Autodesk Inventor part; units mm, degrees
ref_plane "Work Plane1" through (-76.2, 0, 0) normal (-1, 0, 0) x (0, 0, 1)
ref_plane "YZ Plane" through (0, 0, 0) normal (1, 0, 0) x (0, 1, 0)
ref_plane "XZ Plane" through (0, 0, 0) normal (0, 1, 0) x (-1, 0, 0)
sketch "Sketch1" plane through (0, 0, 0) normal (0, 1, 0) x (-1, 0, 0)
  line L0 (0, 0) -> (152.4, 0)
  line L1 (152.4, 0) -> (152.4, 152.4)
  line L2 (152.4, 152.4) -> (0, 152.4)
  line L3 (0, 152.4) -> (0, 0)
  dimension "d0" = 152.4
  dimension "d1" = 152.4
extrude "Extrusion1" add sketch "Sketch1" along normal blind 12.7
hole "Hole1" at (-103.5558, 12.7, 76.2) direction (0, -1, 0) diameter 12.7 end through all
hole "Hole2" at (-50.8, 12.7, 76.2) direction (0, -1, 0) diameter 28.575 end through all
hole "Hole3" at (38.1, 0, 58.6994) direction (0, 1, 0) diameter 4.5 end through all countersink diameter 9.525 countersink angle 82
pattern_circular "Circular Pattern1" count 4 over 360 about axis through (-103.5558, -203.2, 76.2) along (0, 1, 0) of "Hole3"
sketch "Sketch4" plane through (0, 12.7, 0) normal (0, 1, 0) x (1, 0, 0)
  circle A0 centre (-103.5558, -76.2) radius 6.35
  circle A1 centre (-103.5558, -76.2) radius 12.0332
  dimension "d41" = 24.0665
sketch "Sketch5" plane through (0, 12.7, 0) normal (0, 1, 0) x (1, 0, 0)
  circle A0 centre (-50.8, -76.2) radius 14.2875
  circle A1 centre (-103.5558, -76.2) radius 6.35
  line L0 (0, 0) -> (-152.4, 0)
  line L1 (-152.4, 0) -> (-152.4, -152.4)
  line L2 (-152.4, -152.4) -> (0, -152.4)
  line L3 (0, -152.4) -> (0, 0)
  circle A2 centre (-103.5558, -76.2) radius 22.5425
  dimension "d42" = 45.085
extrude "Extrusion4" add sketch "Sketch5" along normal blind 6.35 contours L3 L2 L1 L0
extrude "Extrusion5" cut sketch "Sketch4" against normal blind 2.032
hole "Hole4" at (-26.9748, 0, 76.2) direction (0, 1, 0) diameter 5.08 end through all countersink diameter 9.525 countersink angle 82
pattern_circular "Circular Pattern2" count 6 over 360 about axis through (-50.8, 19.05, 76.2) along (0, -1, 0) of "Hole4"
hole "Hole5" at (0, 9.525, 114.3) direction (-1, 0, 0) diameter 3.9624 depth 38.1 tip angle 118
pattern_linear "Rectangular Pattern1" count 3 spacing 38.1 along (0, 0, -1) of "Hole5"
ref_plane "Work Plane1" through (-76.2, 0, 0) normal (-1, 0, 0) x (0, 0, 1)
mirror "Mirror1" about plane through (-76.2, 0, 0) normal (-1, 0, 0) of "Hole5", "Rectangular Pattern1"
sketch "Sketch6" plane through (0, 19.05, 0) normal (0, 1, 0) x (1, 0, 0)
  circle A0 centre (-11.1125, -11.1125) radius 3.175
  circle A1 centre (-11.1125, -141.2875) radius 3.175
  circle A2 centre (-141.2875, -11.1125) radius 3.175
  circle A3 centre (-141.2875, -141.2875) radius 3.175
  line L0 (0, 0) -> (-152.4, 0)
  line L1 (0, -152.4) -> (0, 0)
  line L2 (-152.4, -152.4) -> (0, -152.4)
  line L3 (-152.4, 0) -> (-152.4, -152.4)
  dimension "d78" = 6.35
  dimension "d79" = 6.35
  dimension "d80" = 6.35
  dimension "d81" = 6.35
  dimension "d82" = 11.1125
  dimension "d83" = 11.1125
  dimension "d84" = 11.1125
  dimension "d85" = 11.1125
  dimension "d86" = 11.1125
  dimension "d87" = 11.1125
  dimension "d88" = 11.1125
  dimension "d89" = 11.1125
extrude "Extrusion6" cut sketch "Sketch6" against normal blind 25.4 contours A0 | A1 | A2 | A3
sketch "Sketch7" plane through (0, 19.05, 0) normal (0, 1, 0) x (1, 0, 0)
  line L0 (0, 0) -> (-152.4, 0)
  line L1 (-152.4, 0) -> (-152.4, -152.4)
  line L2 (0, -152.4) -> (0, 0)
  arc A0 (-127, 0) -> (-25.4, 0) centre (-76.2, 20.5322) ccw
  line L3 (-127, 0) -> (-25.4, 0)
  line L4 (-152.4, -152.4) -> (0, -152.4)
  arc A1 (-25.4, -152.4) -> (-127, -152.4) centre (-76.2, -172.9198) ccw
  line L5 (-152.4, 0) -> (-152.4, -152.4)
  line L6 (0, -152.4) -> (0, 0)
  arc A2 (-152.4, -127) -> (-152.4, -25.4) centre (-210.6083, -76.2) ccw
  arc A3 (0, -25.4) -> (0, -127) centre (58.2083, -76.2) ccw
  line L7 (0, -25.4) -> (0, -127)
  line L8 (-152.4, -25.4) -> (-152.4, -127)
  line L9 (-127, -152.4) -> (-25.4, -152.4)
  line L10 (-152.4, -152.4) -> (0, -152.4)
  dimension "d92" = 25.4
  dimension "d93" = 25.4
  dimension "d94" = 25.4
  dimension "d95" = 25.4
  dimension "d97" = 54.7878
  dimension "d98" = 25.4
  dimension "d99" = 25.4
  dimension "d100" = 25.4
  dimension "d101" = 25.4
extrude "Extrusion7" cut sketch "Sketch7" against normal blind 25.4 contours A0 L0 | L2 A3 | A2 L1 | L4 A1
sketch "Sketch8" plane through (0, 0, 0) normal (0, -1, 0) x (1, 0, 0)
  point P0 (0, 0)
sketch "Sketch9" plane through (0, 0, 0) normal (0, -1, 0) x (1, 0, 0)
  line L0 (-152.4, 25.4) -> (-152.4, 0)
  line L1 (-152.4, 0) -> (-152.4, 25.4)
  line L2 (-152.4, 0) -> (-127, 0)
  line L3 (-127, 0) -> (-152.4, 0)
  line L4 (-127, 0) -> (0, 0)
  line L5 (0, 0) -> (-25.4, 0)
  line L6 (0, 0) -> (0, 25.4)
  line L7 (0, 25.4) -> (0, 0)
  line L8 (0, 25.4) -> (0, 127)
  line L9 (0, 127) -> (0, 152.4)
  line L10 (0, 152.4) -> (0, 127)
  line L11 (0, 152.4) -> (-25.4, 152.4)
  line L12 (-25.4, 152.4) -> (0, 152.4)
  line L13 (-25.4, 152.4) -> (-127, 152.4)
  line L14 (-127, 152.4) -> (-152.4, 152.4)
  line L15 (-152.4, 152.4) -> (-127, 152.4)
  line L16 (-152.4, 152.4) -> (-152.4, 127)
  line L17 (-152.4, 127) -> (-152.4, 152.4)
  line L18 (-152.4, 127) -> (-152.4, 25.4)
  arc A0 (-152.4, 25.4) -> (-152.4, 127) centre (-210.6083, 76.2) ccw
  arc A1 (-152.4, 25.4) -> (-152.4, 127) centre (-210.6083, 76.2) ccw
  arc A2 (-127, 152.4) -> (-25.4, 152.4) centre (-76.2, 172.9198) ccw
  arc A3 (-25.4, 0) -> (-127, 0) centre (-76.2, -20.5322) ccw
  arc A4 (-25.4, 0) -> (-127, 0) centre (-76.2, -20.5322) ccw
  arc A5 (0, 127) -> (0, 25.4) centre (58.2083, 76.2) ccw
extrude "Extrusion8" cut sketch "Sketch9" against normal blind 6.35 contours A0 L16 L14 A2 L11 L9 A5 L6 L4 A3 L2 L0
properties part number "Traveler"
Geometry: final body of the model. Coordinates: model frame, mm. A direction names the side the tool comes from. Give positions to 0.01 mm unless a question says otherwise; leave off trailing zeros. Loops run counter-clockwise (first coordinate to the right, second up) from the corner with the lowest first, then second, coordinate; pieces in that order, holes last. Notation, with made-up numbers: (-14, -22.75) - (-7, -22.75) arc R27 ccw to (-7, 4.25) - close; hole circle Ø2 at (46.5, 66.5). An arc over 180 degrees is marked (long way). Answer as CSV lines item,"result". Start each with the question number.
1. Section B-B, the plane z = 22.5. Return loops of the section in (x, y), plus the area to 3 significant figures.
2. Reachability of faces 1 (the face through (-113, 12.7, 66)), 2 (the face through (-22.25, 8.93, 74.31)), 3 (the face through (-123.704, 7.767, 75.286)) from +Z, -Z, +X, -X, +Y, -Y: full face, straight path, thin tool, end or side. Return the list, or none.
3. Draft query along X for faces 4 (the face through (-64.854, 12.789, 95.468)), 5 (the face through (-77.3, 6.35, 77.3)), 6 (the face through (-152.4, 13, 140)). Return one class per face: released by +X, released by -X, zero draft, split by the parting line, or undercut.
4. Section D-D, the plane z = 44. Return loops of the section in (x, y), plus the area to 3 significant figures.
5. Ray query, L1, parallel to Y at x = -132, z = 114; L2, parallel to X at y = 10.5, z = 76.2; L3, parallel to X at y = 12, z = 139.5. Return the intervals inside material, ascending.
6. Pin query (flat end, axial travel): P1, Ø2.5, axis at y = 9.525, z = 76.2, coming from the +X side; P2, Ø5, axis at y = 13.5, z = 42, coming from the +X side; P3, Ø3, axis at y = 9.525, z = 114.3, coming from the -X side. Return the tip coordinate at first contact, or that it passes through.
7. Section C-C, the plane y = 14.75. Give the number of separate pieces and of enclosed holes in the cut face, plus the area to 3 significant figures.
8. Section A-A, the plane x = -107. Return loops of the section in (y, z).
Answers:
1,outline,"(-152.4, 6.35) - (-110.12, 6.35) - (-110.12, 19.05) - (-152.4, 19.05) - close; (-42.28, 6.35) - (0, 6.35) - (0, 19.05) - (-42.28, 19.05) - close"
1,area,"1,070 mm2"
2,face 1,"+Y"
2,face 2,"+X"
2,face 3,"-X"
3,face 4,"undercut"
3,face 5,"zero draft"
3,face 6,"released by -X"
4,outline,"(-140.38, 6.35) - (-12.02, 6.35) - (-12.02, 19.05) - (-140.38, 19.05) - close"
4,area,"1,630 mm2"
5,L1,"y = 6.35 to 7.57, 11.48 to 19.05"
5,L2,"x = -113.7 to -109.91, -97.21 to -77.17, -72.09 to -65.09"
5,L3,"x = -152.4 to -143.91, -138.66 to -119.61, -32.79 to -13.74, -8.49 to 0"
6,P1,"stops at x = -65.03"
6,P2,"stops at x = -9.78"
6,P3,"stops at x = -114.01"
7,separate pieces,"1"
7,enclosed holes,"12"
7,area,"13,000 mm2"
8,outline,"(6.35, 24.78) - (19.05, 24.78) - (19.05, 53.92) - (12.7, 53.92) - (12.7, 64.67) - (10.67, 64.67) - (10.67, 70.87) - (6.35, 70.87) - close; (6.35, 81.53) - (10.67, 81.53) - (10.67, 87.73) - (12.7, 87.73) - (12.7, 98.48) - (19.05, 98.48) - (19.05, 127.61) - (6.35, 127.61) - close"
